Verification items for the finished model (mm, model axes). Give positions to 0.01 mm unless a question says otherwise; leave off trailing zeros. Order: outer loops, then holes, each group sorted by start corner. A loop starts at its lowest first (then second) coordinate and runs counter-clockwise, first axis right, second up.
(1) Sectioned sample at B-B on z = -58. Record the cut outline in (x, y).
(2) Gauge pin test, flat ends, axial feed: pin 1 (3 mm diameter, centred on y = 6.5, z = 52.5, fed in from -X); pin 2 (1.5 mm diameter, centred on x = 62.5, y = 5, fed in from +Z); pin 3 (1.5 mm diameter, centred on y = 2, z = -30.5, fed in from -X). Record the tip position at first contact, or that the pin passes through.
(3) Sectioned sample at C-C on y = 6.5. Count the separate pieces of the cut face and the enclosed holes in it, plus the area to 3 significant figures.
(4) Sectioned sample at A-A on z = 65. Record the cut outline in (x, y).
(5) Scan lines: L1, parallel to Z at x = -32, y = 9; L2, parallel to X at y = 1, z = 35.5; L3, parallel to Z at x = -24, y = 8.75. Record each from-to range of solid material in increasing order.
(6) Sectioned sample at D-D on z = -34. Record the cut outline in (x, y), plus the area to 3 significant figures.
```python
from build123d import *

# Parameters (mm, degrees)
SKETCH1_R           = 2
SKETCH1_R_2         = 1.65
SKETCH1_R_3         = 2.6
SKETCH1_R_4         = 1
BOSS_EXTRUDE1_DEPTH = 10


with BuildPart() as part:
    # Sketch1 → Boss-Extrude1 (new body)
    with BuildSketch(Plane(origin=(0, 0, 0), x_dir=(1, 0, 0), z_dir=(0, 1, 0))):
        with BuildLine():
            Line((80.08502162, -13.828464902), (66.154165207, 47.206604996))
            ThreePointArc((66.154165207, 47.206604996), (64.22320091, 51.216293675), (60.743723476, 53.991084335))
            Line((60.743723476, 53.991084335), (4.338837391, 81.15424585))
            ThreePointArc((4.338837391, 81.15424585), (0, 82.144557171), (-4.338837391, 81.15424585))
            Line((-4.338837391, 81.15424585), (-60.743723476, 53.991084335))
            ThreePointArc((-60.743723476, 53.991084335), (-64.22320091, 51.216293675), (-66.154165207, 47.206604996))
            Line((-66.154165207, 47.206604996), (-80.08502162, -13.828464902))
            ThreePointArc((-80.08502162, -13.828464902), (-80.08502162, -18.278883581), (-78.154057323, -22.28857226))
            Line((-78.154057323, -22.28857226), (-39.120665047, -71.234898019))
            ThreePointArc((-39.120665047, -71.234898019), (-35.641187614, -74.009688679), (-31.302350222, -75))
            Line((-31.302350222, -75), (31.302350222, -75))
            ThreePointArc((31.302350222, -75), (35.641187614, -74.009688679), (39.120665047, -71.234898019))
            Line((39.120665047, -71.234898019), (78.154057323, -22.28857226))
            ThreePointArc((78.154057323, -22.28857226), (80.08502162, -18.278883581), (80.08502162, -13.828464902))
        make_face()
        with Locations(Location((-31.302350222, -65, 0), (0, 0, 270))):
            Circle(SKETCH1_R, mode=Mode.SUBTRACT)
        with Locations(Location((70.335742498, -16.053674242, 0), (0, 0, 270))):
            Circle(SKETCH1_R, mode=Mode.SUBTRACT)
        with Locations(Location((0, 72.144557171, 0), (0, 0, 270))):
            Circle(SKETCH1_R, mode=Mode.SUBTRACT)
        with Locations(Location((56.404886085, 44.981395656, 0), (0, 0, 270))):
            Circle(SKETCH1_R, mode=Mode.SUBTRACT)
        with Locations(Location((-56.404886085, 44.981395656, 0), (0, 0, 270))):
            Circle(SKETCH1_R, mode=Mode.SUBTRACT)
        with Locations(Location((-70.335742498, -16.053674242, 0), (0, 0, 270))):
            Circle(SKETCH1_R, mode=Mode.SUBTRACT)
        with Locations(Location((31.302350222, -65, 0), (0, 0, 270))):
            Circle(SKETCH1_R, mode=Mode.SUBTRACT)
        with Locations(Location((-20, -48, 0), (0, 0, 270))):
            Circle(SKETCH1_R_2, mode=Mode.SUBTRACT)
        with Locations(Location((-20, -36, 0), (0, 0, 270))):
            Circle(SKETCH1_R_2, mode=Mode.SUBTRACT)
        with Locations(Location((-22.633605309, -7.531262225, 0), (0, 0, 270))):
            Circle(SKETCH1_R_3, mode=Mode.SUBTRACT)
        with Locations(Location((2.305986765, 23.741997074, 0), (0, 0, 270))):
            Circle(SKETCH1_R_3, mode=Mode.SUBTRACT)
        with Locations(Location((-7.531262225, 22.633605309, 0), (0, 0, 270))):
            Circle(SKETCH1_R_3, mode=Mode.SUBTRACT)
        with Locations(Location((23.741997074, -2.305986765, 0), (0, 0, 270))):
            Circle(SKETCH1_R_3, mode=Mode.SUBTRACT)
        with Locations(Location((41.476576253, -58.657425978, 0), (0, 0, 270))):
            Circle(SKETCH1_R_4, mode=Mode.SUBTRACT)
        with Locations(Location((66.416168327, -27.384166679, 0), (0, 0, 270))):
            Circle(SKETCH1_R_4, mode=Mode.SUBTRACT)
        with Locations(Location((46.870381266, -11.796921632, 0), (0, 0, 270))):
            Circle(SKETCH1_R_4, mode=Mode.SUBTRACT)
        with Locations(Location((21.930789191, -43.070180931, 0), (0, 0, 270))):
            Circle(SKETCH1_R_4, mode=Mode.SUBTRACT)
        Polygon((0.316683361, -2.810642569), (2.810642569, 0.316683361), (-0.316683361, 2.810642569), (-2.810642569, -0.316683361), align=None, mode=Mode.SUBTRACT)
    extrude(amount=BOSS_EXTRUDE1_DEPTH)


solid = part.part
```
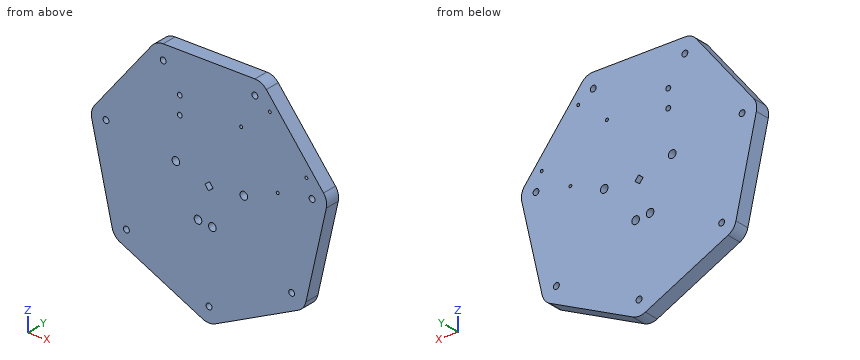
Ans:
1. outline: (-52.42, 0) - (52.42, 0) - (52.42, 10) - (-52.42, 10) - close
2. pin 1: stops at x = -55.26
2. pin 2: stops at z = 42.86
2. pin 3: stops at x = -70.14
3. separate pieces: 1
3. enclosed holes: 18
3. area: 18,700 mm2
4. outline: (-44.09, 0) - (-33.3, 0) - (-33.3, 10) - (-44.09, 10) - close; (-29.3, 0) - (29.3, 0) - (29.3, 10) - (-29.3, 10) - close; (33.3, 0) - (44.09, 0) - (44.09, 10) - (33.3, 10) - close
5. L1: z = -67.83 to 63.13, 66.87 to 74.98
5. L2: x = -67.62 to -21.57, -18.43 to 67.62
5. L3: z = -71.69 to 5.32, 9.74 to 75
6. outline: (-69.17, 0) - (69.17, 0) - (69.17, 10) - (-69.17, 10) - close
6. area: 1,380 mm2
